Design review of the part shown in the three views and the two pictorial views. Dimensions are in mm from the part's minimum x, y and z. A direction names the side the tool comes from. Round coordinates to 2 decimals unless told otherwise and drop trailing zeros. Loops run counter-clockwise (first coordinate to the right, second up) from the corner with the lowest first, then second, coordinate; pieces in that order, holes last. Notation, with made-up numbers: M -27,85 L -12,85 A9 cw -12,95 Z; hole C -34.5,75.5 d8. An arc over 180 degrees is marked long. Answer in a Markdown table with one row per item. Add a question column.
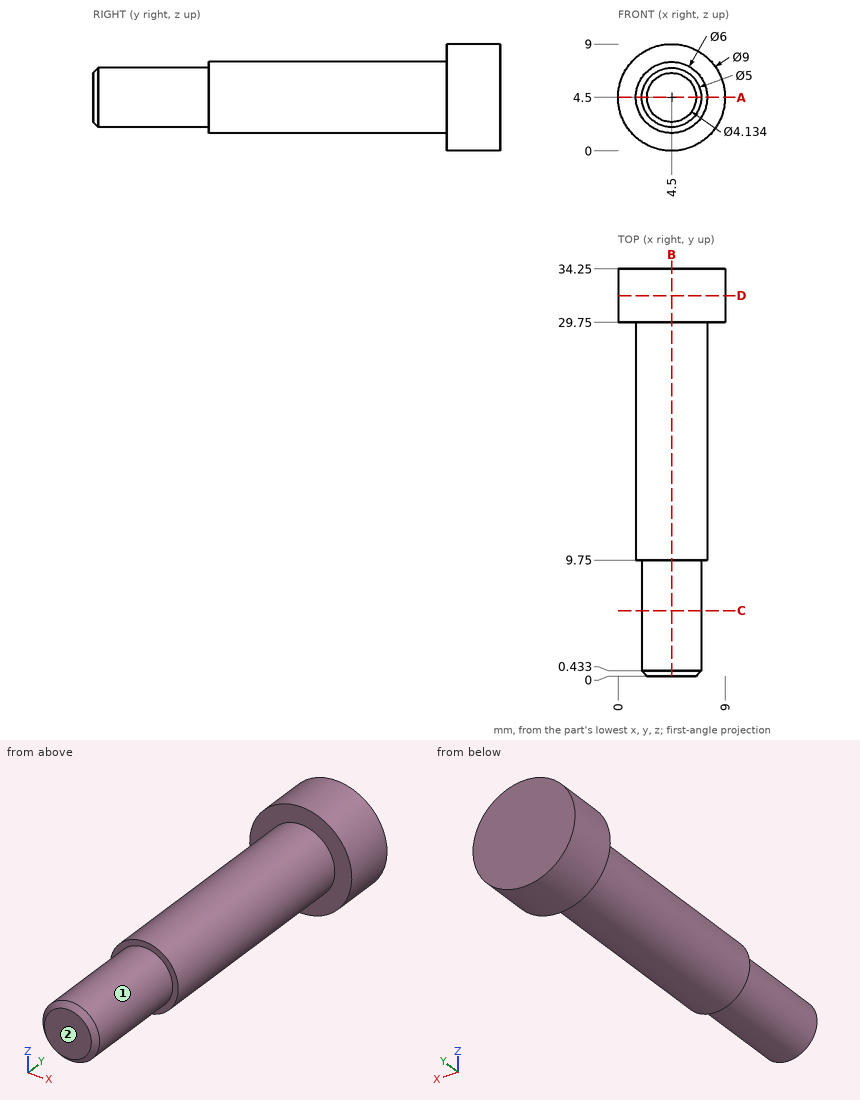
1. For pin 1 Ø2 at (x, y) = (4.5, 21) entering from +Z; pin 2 Ø5 at (y, z) = (9, 7.5) entering from -X, all flat-tipped, find the tip position at first contact; note any pin that passes through.
2. Take a section at D-D, the plane y = 32. State the section outline as (x, z) points, and give its area (3 significant figures).
3. Take a section at B-B, the plane x = 4.5. State the section outline as (y, z) points, and give its area (3 significant figures).
4. Take a section at A-A, the plane z = 4.5. State the section outline as (x, y) points, and give its area (3 significant figures).
5. Take a section at C-C, the plane y = 5.5. State the section outline as (x, z) points.
6. Machinability: for the marked faces 1 and 2, which of the approach directions +Z, -Z, +X, -X, +Y, -Y give a long, thin tool a straight path to every point of the face, cutting with its end or side? Answer none if there is none.
7. To check wall thickness, follow probe 1 along Y at (x, z) = (8, 7); probe 2 along Z at (x, y) = (4.75, 32.5); probe 3 along X at (y, z) = (25.5, 3.5). State the ranges of each line that lie inside material, in increasing order.
Check sheet entries:
| question | item | result |
|---|---|---|
| 1 | pin 1 | stops at z = 7.5 |
| 1 | pin 2 | stops at x = 1.56 |
| 2 | outline | C 4.5,4.5 d9 |
| 2 | area | 63.6 mm^2 |
| 3 | outline | M 0,2.43 L 0.43,2 L 9.75,2 L 9.75,1.5 L 29.75,1.5 L 29.75,0 L 34.25,0 L 34.25,9 L 29.75,9 L 29.75,7.5 L 9.75,7.5 L 9.75,7 L 0.43,7 L 0,6.57 Z |
| 3 | area | 209 mm^2 |
| 4 | outline | M 0,29.75 L 1.5,29.75 L 1.5,9.75 L 2,9.75 L 2,0.43 L 2.43,0 L 6.57,0 L 7,0.43 L 7,9.75 L 7.5,9.75 L 7.5,29.75 L 9,29.75 L 9,34.25 L 0,34.25 Z |
| 4 | area | 209 mm^2 |
| 5 | outline | C 4.5,4.5 d5 |
| 6 | face 1 | -Y |
| 6 | face 2 | +Z, -Z, +X, -X, -Y |
| 7 | probe 1 | y = 29.75 to 34.25 |
| 7 | probe 2 | z = 0.01 to 8.99 |
| 7 | probe 3 | x = 1.67 to 7.33 |
